Work out the finished part from the listing and answer in its coordinate system (mm). Face numbers are marked on the shaded views. A direction names the side the tool comes from. Round coordinates to 2 decimals unless told otherwise and drop trailing zeros. Loops run counter-clockwise (first coordinate to the right, second up) from the corner with the lowest first, then second, coordinate; pieces in that order, holes last.
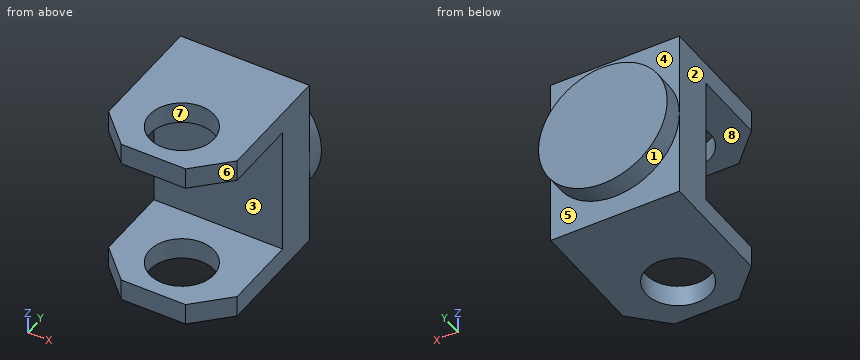
```python
from build123d import *

# Parameters (mm, degrees)
F2_DEPTH = 19.05
F3_R     = 9.525
F4_DEPTH = 50.801
F5_SIZE  = 9.525
F0_R     = 19.05
F6_DEPTH = 12.7


with BuildPart() as f2:
    # F1 (on Right) → F2 (new body, symmetric)
    with BuildSketch(Plane.YZ):
        Polygon((-38.1, -19.05), (-38.1, -25.4), (6.7289513536, -25.4), (6.7289513536, 25.4), (-38.1, 25.4), (-38.1, 19.05), (-6.35, 19.05), (-6.35, -19.05), align=None)
    extrude(amount=F2_DEPTH, both=True)

    # F3 (on face) → F4 (cut, through all)
    with BuildSketch(Plane(origin=(0, 0, -25.4), x_dir=(1, 0, 0), z_dir=(0, 0, -1))):
        with Locations((0, 24.1716690361)):
            Circle(F3_R)
    extrude(amount=-F4_DEPTH, mode=Mode.SUBTRACT)

    # F5
    f5_edges = [f2.edges().sort_by_distance(p)[0] for p in [
        (-19.05, -38.1, 22.225),
        (19.05, -38.1, 22.225),
        (-19.05, -38.1, -22.225),
        (19.05, -38.1, -22.225),
    ]]
    chamfer(f5_edges, length=F5_SIZE)

    # F0 (on Front) → F6 (join)
    with BuildSketch(Plane.XZ):
        Circle(F0_R)
    extrude(amount=-F6_DEPTH)


solid = f2.part
```
1. Find section C-C (y = -25). Write down the section's boundary in (x, z), then the cut area to 3 significant figures.
Answer key:
outline: (-19.05, -25.4) - (-9.49, -25.4) - (-9.49, -19.05) - (-19.05, -19.05) - close; (-19.05, 19.05) - (-9.49, 19.05) - (-9.49, 25.4) - (-19.05, 25.4) - close; (9.49, -25.4) - (19.05, -25.4) - (19.05, -19.05) - (9.49, -19.05) - close; (9.49, 19.05) - (19.05, 19.05) - (19.05, 25.4) - (9.49, 25.4) - close
area: 243 mm2
2. Which of the six approach directions +Z, -Z, +X, -X, +Y, -Y give full straight-line access (tool end or side, diameter ignored) to the marked faces 1, 2, 3, 4 and 5?
Answer key:
face 1: +Y
face 2: +Z, -Z, -X, +Y, -Y
face 3: +X, -X, -Y
face 4: +Z, +Y
face 5: -Z, +Y
3. Find section B-B (y = -13). Write down the section's boundary in (x, z).
Answer key:
outline: (-19.05, -25.4) - (19.05, -25.4) - (19.05, -19.05) - (-19.05, -19.05) - close; (-19.05, 19.05) - (19.05, 19.05) - (19.05, 25.4) - (-19.05, 25.4) - close
4. Given pin 1 (10 mm diameter, centred on x = 6.5, z = -4, fed in from -Y), flat-ended and moving along its own axis, determine where the tip first touches the part or whether it passes through.
Answer key:
pin 1: stops at y = -6.35
5. Find section A-A (x = 0). Write down the section's boundary in (y, z), then the cut area to 3 significant figures.
Answer key:
outline: (-38.1, -25.4) - (-33.7, -25.4) - (-33.7, -19.05) - (-38.1, -19.05) - close; (-38.1, 19.05) - (-33.7, 19.05) - (-33.7, 25.4) - (-38.1, 25.4) - close; (-14.65, -25.4) - (6.73, -25.4) - (6.73, -19.05) - (12.7, -19.05) - (12.7, 19.05) - (6.73, 19.05) - (6.73, 25.4) - (-14.65, 25.4) - (-14.65, 19.05) - (-6.35, 19.05) - (-6.35, -19.05) - (-14.65, -19.05) - close
area: 1,050 mm2
6. Determine the mould class of the marked faces 6, 7 and 8 for opening direction X: +X half, -X half, draft (parallel to the pull), parting line (faces both ways), or undercut.
Answer key:
face 6: +X half
face 7: undercut
face 8: draft
7. Find section D-D (z = -10). Write down the section's boundary in (x, y).
Answer key:
outline: (-19.05, -6.35) - (19.05, -6.35) - (19.05, 6.73) - (16.21, 6.73) - (16.21, 12.7) - (-16.21, 12.7) - (-16.21, 6.73) - (-19.05, 6.73) - close
8. Consider probe 1 along Y at (x, z) = (0, 23); probe 2 along Z at (x, y) = (-17, -19). Determine where each line is inside the solid, lowest interval first.
Answer key:
probe 1: y = -38.1 to -33.7, -14.65 to 6.73
probe 2: z = -25.4 to -19.05, 19.05 to 25.4
